Here's how the part is built. I have some questions about the finished solid (model axes, mm). Face numbers are marked on the shaded views. A direction names the side the tool comes from. Give positions to 0.01 mm unless a question says otherwise; leave off trailing zeros. Write each loop counter-clockwise with the first axis right and the second up, starting at its lowest first coordinate (ties: lowest second). Pieces come first, ordered by that corner, then holes. Notation, with made-up numbers: (47, 49.25) -> (71, 49.25) arc R15 ccw to (71, 70.25) -> close; hole circle Ø8 at (-21.5, 32.5). An arc over 180 degrees is marked (long way). Return JSON: item names as keys, results as strings.
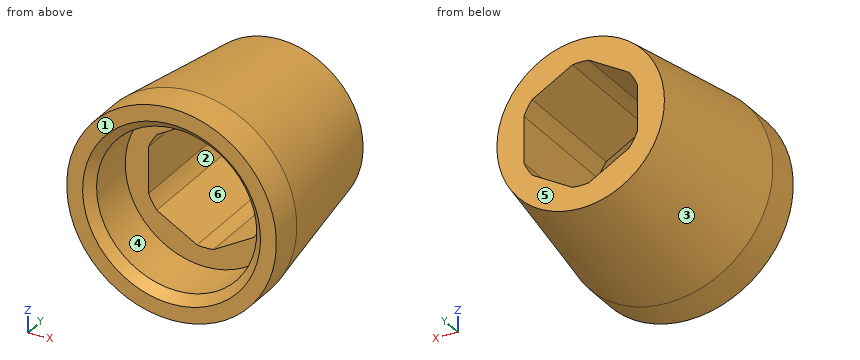
from build123d import *

# Parameters (mm, degrees)
BOSS_EXTRUDE1_START = -10.876
BOSS_EXTRUDE1_DEPTH = 10.876
CHAMFER1_SIZE       = 0.75


with BuildPart() as part:
    # Sketch1 → Revolve1 (revolve)
    with BuildSketch(Plane.XY, mode=Mode.PRIVATE) as revolve1_sk:
        Polygon((6.8, 0), (6.8, 4.953), (5.2, 4.953), (5.2, 15.829), (7.112, 15.829), (8.9, 3), (8.9, 0), align=None)
    revolve(revolve1_sk.sketch.rotate(Axis((0, 0, 0), (0, 1, 0)), 90), axis=Axis((0, 0, 0), (0, 1, 0)))

    # Sketch4 → Boss-Extrude1 (add)
    with BuildSketch(Plane.XZ.offset(-4.953).offset(BOSS_EXTRUDE1_START)):
        with BuildLine():
            Line((0.700412138, 5.152613205), (4.112087862, 3.182881307))
            ThreePointArc((4.112087862, 3.182881307), (2.6, 4.5033321), (0.700412138, 5.152613205))
        make_face()
        with BuildLine():
            ThreePointArc((4.8125, -1.969731898), (5.2, 0), (4.8125, 1.969731898))
            Line((4.8125, 1.969731898), (4.8125, -1.969731898))
        make_face()
        with BuildLine():
            Line((-4.112087862, 3.182881307), (-0.700412138, 5.152613205))
            ThreePointArc((-0.700412138, 5.152613205), (-2.6, 4.5033321), (-4.112087862, 3.182881307))
        make_face()
        with BuildLine():
            ThreePointArc((0.700412138, -5.152613205), (2.6, -4.5033321), (4.112087862, -3.182881307))
            Line((4.112087862, -3.182881307), (0.700412138, -5.152613205))
        make_face()
        with BuildLine():
            Line((-4.8125, -1.969731898), (-4.8125, 1.969731898))
            ThreePointArc((-4.8125, 1.969731898), (-5.2, 0), (-4.8125, -1.969731898))
        make_face()
        with BuildLine():
            ThreePointArc((-4.112087862, -3.182881307), (-2.6, -4.5033321), (-0.700412138, -5.152613205))
            Line((-0.700412138, -5.152613205), (-4.112087862, -3.182881307))
        make_face()
    extrude(amount=BOSS_EXTRUDE1_DEPTH)

    # Chamfer1
    chamfer1_edges = [part.edges().sort_by_distance(p)[0] for p in [
        (0, 0, 6.8),
    ]]
    chamfer(chamfer1_edges, length=CHAMFER1_SIZE)


solid = part.part
1. If we mould it in two halves opening along X, with no side actions, what happens to the marked faces 1, 2 and 3? For each: released by +X, released by -X, zero draft, split by the parting line, or undercut.
Taken from the geometry:
{"face 1": "zero draft", "face 2": "undercut", "face 3": "split by the parting line"}
2. For pin 1 Ø6 at (y, z) = (8, 0.5) entering from -X; pin 2 Ø7 at (x, z) = (0.5, 2) entering from -Y; pin 3 Ø2 at (x, y) = (6.5, 10) entering from -Z, each with a flat end and sliding along its axis, tell me the tip position at first contact or that it passes through.
Taken from the geometry:
{"pin 1": "stops at x = -8.62", "pin 2": "stops at y = 4.95", "pin 3": "stops at z = -5.72"}
3. Which directions (+Z, -Z, +X, -X, +Y, -Y) give clear straight access to the entire face, cutting with the end or side of a thin tool? Please do the marked faces 4, 5 and 6.
Taken from the geometry:
{"face 4": "-Y", "face 5": "+Z, -Z, +X, -X, +Y", "face 6": "+Y, -Y"}
4. Suppose I cut it at A-A, the plane x = 0. List the corners of the cut face in (y, z) for me.
Taken from the geometry:
{"outline": "(0, -8.9) -> (3, -8.9) -> (15.83, -7.11) -> (15.83, -5.2) -> (4.95, -5.2) -> (4.95, -6.8) -> (0.75, -6.8) -> (0, -7.55) -> close; (0, 7.55) -> (0.75, 6.8) -> (4.95, 6.8) -> (4.95, 5.2) -> (15.83, 5.2) -> (15.83, 7.11) -> (3, 8.9) -> (0, 8.9) -> close"}
5. If I drill on line 1 (X direction, y = 2.05, z = 0); line 2 (X direction, y = 2.75, z = 4); line 3 (Z direction, x = -0.75, y = 11.25), over which ranges is the centre line in solid material (lowest first)? Write a range as [from, to].
Taken from the geometry:
{"line 1": "x = [-8.9, -6.8], [6.8, 8.9]", "line 2": "x = [-7.95, -5.5], [5.5, 7.95]", "line 3": "z = [-7.71, -5.12], [5.12, 7.71]"}
6. Suppose I cut it at B-B, the plane z = 0. List the corners of the cut face in (x, y) for me.
Taken from the geometry:
{"outline": "(-8.9, 0) -> (-7.55, 0) -> (-6.8, 0.75) -> (-6.8, 4.95) -> (-4.81, 4.95) -> (-4.81, 15.83) -> (-7.11, 15.83) -> (-8.9, 3) -> close; (4.81, 4.95) -> (6.8, 4.95) -> (6.8, 0.75) -> (7.55, 0) -> (8.9, 0) -> (8.9, 3) -> (7.11, 15.83) -> (4.81, 15.83) -> close"}
7. Suppose I cut it at D-D, the plane y = 7.5. List the corners of the cut face in (x, z) for me, and give its area (3 significant figures).
Taken from the geometry:
{"outline": "circle Ø16.55 at (0, 0); hole (-4.81, -1.97) arc R5.2 ccw to (-4.11, -3.18) -> (-0.7, -5.15) arc R5.2 ccw to (0.7, -5.15) -> (4.11, -3.18) arc R5.2 ccw to (4.81, -1.97) -> (4.81, 1.97) arc R5.2 ccw to (4.11, 3.18) -> (0.7, 5.15) arc R5.2 ccw to (-0.7, 5.15) -> (-4.11, 3.18) arc R5.2 ccw to (-4.81, 1.97) -> close", "area": "136 mm²"}
8. Suppose I cut it at C-C, the plane y = 13. List the corners of the cut face in (x, z) for me, and give its area (3 significant figures).
Taken from the geometry:
{"outline": "circle Ø15.01 at (0, 0); hole (-4.81, -1.97) arc R5.2 ccw to (-4.11, -3.18) -> (-0.7, -5.15) arc R5.2 ccw to (0.7, -5.15) -> (4.11, -3.18) arc R5.2 ccw to (4.81, -1.97) -> (4.81, 1.97) arc R5.2 ccw to (4.11, 3.18) -> (0.7, 5.15) arc R5.2 ccw to (-0.7, 5.15) -> (-4.11, 3.18) arc R5.2 ccw to (-4.81, 1.97) -> close", "area": "98.2 mm²"}
